The model under review builds one solid part; all positions refer to its coordinate system, in mm. A direction names the side the tool comes from. Give positions to 0.01 mm unless a question says otherwise; leave off trailing zeros. Order: outer loops, then holes, each group sorted by start corner. A loop starts at its lowest first (then second) coordinate and runs counter-clockwise, first axis right, second up. Notation, with made-up numbers: (38.25, 74) - (54.25, 74) arc R16 cw to (54.25, 93) - close; hole circle Ø4 at (69, 69). An arc over 180 degrees is marked (long way). Write item = value, one per line. Start each with the question number.
1. For P1, Ø9, axis at x = -2.5, y = 33.5, coming from the +Z side; P2, Ø1.5, axis at y = 31.5, z = -2, coming from the -X side; P3, Ø5, axis at x = 0, y = 6, coming from the -Z side, all flat-tipped, find the tip position at first contact; note any pin that passes through.
2. Machinability: for faces 4 (the flat face through (12.5, 4, 0)), 5 (the cylindrical face through (-10.836, -1.479, -6.87)), 6 (the flat face through (0, 32, -11)), which of the approach directions +Z, -Z, +X, -X, +Y, -Y give a long, thin tool a straight path to every point of the face, cutting with its end or side? Answer none if there is none.
3. Mouldability with a two-part tool opening along X and no side actions: class faces 1 (the flat face through (-10, -3, -7)), 2 (the cylindrical face through (-10.836, -1.479, 7.13)), 3 (the flat face through (-15, 18, 0)) as pulls with the +X half, pulls with the -X half, needs draft (parallel to the pull), parting line crosses it, or undercut.
4. Wall thickness on probe 1 along Y at (x, z) = (8.5, -3.5); probe 2 along Y at (x, z) = (12, 9.5); probe 3 along Z at (x, y) = (11, 0.5): over which ranges is each line inside the solid? List them lowest first.
5. We need section C-C, the plane x = 10.25. Give the boundary of the cut face in (y, z).
6. We need section B-B, the plane z = 0. Give the boundary of the cut face in (x, y), and give its area (3 significant figures).
7. We need section A-A, the plane x = -1.75. Give the boundary of the cut face in (y, z).
8. We need section D-D, the plane z = 7. Give the boundary of the cut face in (x, y), and give its area (3 significant figures).
from build123d import *

# Parameters (mm, degrees)
SKETCH_1_W      = 25
SKETCH_1_H      = 22
EXTRUDE_1_DEPTH = 9
SKETCH_2_W      = 19
SKETCH_2_H      = 22
EXTRUDE_2_DEPTH = 27
SKETCH_4_R      = 0.6
EXTRUDE_4_DEPTH = 3
SKETCH_3_W      = 30
SKETCH_3_H      = 35
SKETCH_3_W_2    = 19
SKETCH_3_H_2    = 22
EXTRUDE_6_DEPTH = 19


with BuildPart() as part:
    # Эскиз1 → Бобышка-Вытянуть1 (new body)
    with BuildSketch(Plane(origin=(0, 0, 0), x_dir=(1, 0, 0), z_dir=(0, 1, 0))):
        Rectangle(SKETCH_1_W, SKETCH_1_H)
    extrude(amount=EXTRUDE_1_DEPTH)

    # Эскиз2 → Бобышка-Вытянуть2 (add)
    with BuildSketch(Plane(origin=(0, 9, 0), x_dir=(1, 0, 0), z_dir=(0, 1, 0))):
        Rectangle(SKETCH_2_W, SKETCH_2_H)
    extrude(amount=EXTRUDE_2_DEPTH)

    # Эскиз4 → Бобышка-Вытянуть4 (add)
    with BuildSketch(Plane.XZ):
        with Locations(Location((10.25, -7, 0), (0, 0, 270))):
            Circle(SKETCH_4_R)
        with Locations(Location((10.25, 7, 0), (0, 0, 270))):
            Circle(SKETCH_4_R)
        with Locations(Location((-10.25, 7, 0), (0, 0, 270))):
            Circle(SKETCH_4_R)
        with Locations(Location((-10.25, -7, 0), (0, 0, 270))):
            Circle(SKETCH_4_R)
        with Locations(Location((-10.25, 0, 0), (0, 0, 270))):
            Circle(SKETCH_4_R)
    extrude(amount=EXTRUDE_4_DEPTH)

    # Эскиз3 → Бобышка-Вытянуть6 (add)
    with BuildSketch(Plane(origin=(0, 9, 0), x_dir=(1, 0, 0), z_dir=(0, 1, 0))):
        Rectangle(SKETCH_3_W, SKETCH_3_H)
        Rectangle(SKETCH_3_W_2, SKETCH_3_H_2, mode=Mode.SUBTRACT)
    extrude(amount=EXTRUDE_6_DEPTH)


solid = part.part
Model answer:
q1.P1 = 11
q1.P2 = -9.5
q1.P3 = -11
q2.face_4 = +Z, -Z, +X, -Y
q2.face_5 = -Y
q2.face_6 = -Z, +X, -X, +Y
q3.face_1 = needs draft
q3.face_2 = undercut
q3.face_3 = pulls with the -X half
q4.probe_1 = 0 to 36
q4.probe_2 = 0 to 28
q4.probe_3 = -11 to 11
q5.outline = (-3, -7.6) - (0, -7.6) - (0, -11) - (9, -11) - (9, -17.5) - (28, -17.5) - (28, 17.5) - (9, 17.5) - (9, 11) - (0, 11) - (0, 7.6) - (-3, 7.6) - (-3, 6.4) - (0, 6.4) - (0, -6.4) - (-3, -6.4) - close
q6.outline = (-15, 9) - (-12.5, 9) - (-12.5, 0) - (-10.85, 0) - (-10.85, -3) - (-9.65, -3) - (-9.65, 0) - (12.5, 0) - (12.5, 9) - (15, 9) - (15, 28) - (9.5, 28) - (9.5, 36) - (-9.5, 36) - (-9.5, 28) - (-15, 28) - close
q6.area = 951 mm2
q7.outline = (0, -11) - (9, -11) - (9, -17.5) - (28, -17.5) - (28, -11) - (36, -11) - (36, 11) - (28, 11) - (28, 17.5) - (9, 17.5) - (9, 11) - (0, 11) - close
q8.outline = (-15, 9) - (-12.5, 9) - (-12.5, 0) - (-10.85, 0) - (-10.85, -3) - (-9.65, -3) - (-9.65, 0) - (9.65, 0) - (9.65, -3) - (10.85, -3) - (10.85, 0) - (12.5, 0) - (12.5, 9) - (15, 9) - (15, 28) - (9.5, 28) - (9.5, 36) - (-9.5, 36) - (-9.5, 28) - (-15, 28) - close
q8.area = 954 mm2
